Geometry: final body of the model. Coordinates: model frame, mm. A direction names the side the tool comes from. Coordinates: 2 decimals unless noted, no trailing zeros. Loops run counter-clockwise (first coordinate to the right, second up) from the corner with the lowest first, then second, coordinate; pieces in that order, holes last. Notation, with made-up numbers: M 57,27 L 95,27 A21 cw 95,31 Z; hole C 45,22 d2. An arc over 180 degrees is marked long. Write item = value, one per line. Start each with the question number.
```python
from build123d import *

# Parameters (mm, degrees)
F0_R     = 3.175
F1_DEPTH = 2.38125
F3_D     = 1.9939
F3_DEPTH = 8.73225


with BuildPart() as f1:
    # F0 (on Front) → F1 (new body, symmetric)
    with BuildSketch(Plane.XZ):
        with BuildLine():
            Line((-5.8666350314, 2.4300397955), (-8.0666231682, 3.3413047188))
            ThreePointArc((-8.0666231682, 3.3413047188), (0, -8.73125), (8.0666231682, 3.3413047188))
            Line((8.0666231682, 3.3413047188), (5.8666350314, 2.4300397955))
            ThreePointArc((5.8666350314, 2.4300397955), (0, 6.35), (-5.8666350314, 2.4300397955))
        make_face()
        Circle(F0_R, mode=Mode.SUBTRACT)
    extrude(amount=F1_DEPTH, both=True)

    # F3 (through all, one way)
    with BuildSketch(Plane.XY):
        with Locations((0, 0)):
            Circle(F3_D / 2)
    extrude(amount=-F3_DEPTH, mode=Mode.SUBTRACT)


solid = f1.part
```
Item 1: Section query A-A (z = 0). Return the cut outline in (x, y) (3 decimals).
Item 2: Line query: line 1 (Y direction, x = 0, z = -5.8); line 2 (Z direction, x = 0, y = 0.2) (3 decimals); line 3 (X direction, y = -0.1, z = 2). Output: solid intervals per line, ascending. Write a range as from..to.
Item 3: First-contact query: pin 1 (1 mm diameter, centred on y = -1, z = 0.5, fed in from -X). Flat tip, straight axial feed; report the tip coordinate or a pass-through.
Item 4: Reachability of faces 1 (the flat face through (7, 0, 2.9)), 2 (the cylindrical face through (0.95, 0.3, -5.83)), 3 (the flat face through (2, 2.381, -3)) from +Z, -Z, +X, -X, +Y, -Y: full face, straight path, thin tool, end or side. Return the list, or none.
Item 5: Pull-direction query (X, two-part tool) for faces 4 (the cylindrical face through (-0.24, -1.621, -8.728)), 5 (the flat face through (2, -2.381, -3)), 6 (the flat face through (-7, 0, 2.9)); classes: released by +X, released by -X, zero draft, split by the parting line, or undercut.
Item 6: Section query B-B (x = 0). Return the cut outline in (y, z) (3 decimals), plus the area to 3 significant figures.
Verdict:
q1.outline = M -8.731,-2.381 L -3.175,-2.381 L -3.175,2.381 L -8.731,2.381 Z; M 3.175,-2.381 L 8.731,-2.381 L 8.731,2.381 L 3.175,2.381 Z
q2.line_1 = -2.38..-1, 1..2.38
q2.line_2 = 3.175..6.35
q2.line_3 = -8.5..-2.47, 2.47..8.5
q3.pin_1 = -8.73
q4.face_1 = +Z, +Y, -Y
q4.face_2 = -Z
q4.face_3 = +Z, -Z, +X, -X, +Y
q5.face_4 = split by the parting line
q5.face_5 = zero draft
q5.face_6 = undercut
q6.outline = M -2.381,-8.731 L -0.997,-8.731 L -0.997,-3.175 L -2.381,-3.175 Z; M -2.381,3.175 L 2.381,3.175 L 2.381,6.35 L -2.381,6.35 Z; M 0.997,-8.731 L 2.381,-8.731 L 2.381,-3.175 L 0.997,-3.175 Z
q6.area = 30.5 mm2
